from build123d import *

# Parameters (mm, degrees)
SKETCH1_R           = 85
SKETCH1_R_2         = 8.5
BOSS_EXTRUDE1_DEPTH = 10
SKETCH2_R           = 8.5
CUT_EXTRUDE1_DEPTH  = 10
SKETCH4_R           = 5
CUT_EXTRUDE3_DEPTH  = 60


with BuildPart() as part:
    # Sketch1 → Boss-Extrude1 (new body)
    with BuildSketch(Plane.XY):
        Circle(SKETCH1_R)
        Circle(SKETCH1_R_2, mode=Mode.SUBTRACT)
    extrude(amount=BOSS_EXTRUDE1_DEPTH)

    # Sketch2 → Cut-Extrude1 (cut)
    with BuildSketch(Plane.XY.offset(10)):
        with Locations((0, 60)):
            Circle(SKETCH2_R)
        with Locations((57.063390978, 18.541019662)):
            Circle(SKETCH2_R)
        with Locations((35.267115138, -48.541019662)):
            Circle(SKETCH2_R)
        with Locations((-35.267115138, -48.541019662)):
            Circle(SKETCH2_R)
        with Locations((-57.063390978, 18.541019662)):
            Circle(SKETCH2_R)
    extrude(amount=-CUT_EXTRUDE1_DEPTH, mode=Mode.SUBTRACT)

    # Sketch4 → Cut-Extrude3 (cut)
    with BuildSketch(Plane.XY.offset(10)):
        with Locations((0, -48)):
            Circle(SKETCH4_R)
    extrude(amount=-CUT_EXTRUDE3_DEPTH, mode=Mode.SUBTRACT)


solid = part.part
Model file for the job. Use its own axes, mm. Give positions to 0.01 mm unless a question says otherwise; leave off trailing zeros. Order: outer loops, then holes, each group sorted by start corner. A loop starts at its lowest first (then second) coordinate and runs counter-clockwise, first axis right, second up. Notation, with made-up numbers: M -9.5,7.25 L 15.5,7.25 A14 ccw 15.5,16.25 Z; hole C -30.5,-3 d11. An arc over 180 degrees is marked long. Put each result on its own line as item: value. Start each with the question number.
(1) Pin check, flat tips, straight feed: pin 1 Ø1.5 at (y, z) = (36.5, 8.5) entering from +X; pin 2 Ø6 at (y, z) = (37.5, 5.5) entering from -X; pin 3 Ø5 at (x, z) = (46.5, 6.5) entering from +Y. Stop position of each tip, or through.
(2) Band-saw the part on D-D on z = 3. Give the cut face in (x, y).
(3) Band-saw the part on B-B on y = 54. Give the cut face in (x, z), then the cut area to 3 significant figures.
(4) Band-saw the part on A-A on x = 0. Give the cut face in (y, z).
(5) Pull direction Y, two halves, no side cores. Call faces 1 (the face through (-67.453, -51.721, 4.93)), 2 (the face through (-49.21, 15.29, 5.07)), 3 (the face through (18, 1, 0)): released by +Y, released by -Y, zero draft, split by the parting line, or undercut.
(6) Drill centre lines: L1, parallel to Y at x = -0.5, z = 6.75; L2, parallel to Y at x = -32.5, z = 7.25; L3, parallel to X at y = 65, z = 4.25. Where is each one in solid material? Low to high. Write a range as [from, to].
(7) Band-saw the part on C-C on x = 56. Give the cut face in (y, z), then the cut area to 3 significant figures.
Results below:
1. pin 1: stops at x = 77.12
1. pin 2: stops at x = -77.68
1. pin 3: stops at y = 72.73
2. outline: C 0,0 d170; hole C -57.06,18.54 d17; hole C -35.27,-48.54 d17; hole C 0,0 d17; hole C 0,60 d17; hole C 0,-48 d10; hole C 35.27,-48.54 d17; hole C 57.06,18.54 d17
3. outline: M -65.64,0 L -6.02,0 L -6.02,10 L -65.64,10 Z; M 6.02,0 L 65.64,0 L 65.64,10 L 6.02,10 Z
3. area: 1,190 mm2
4. outline: M -85,0 L -53,0 L -53,10 L -85,10 Z; M -43,0 L -8.5,0 L -8.5,10 L -43,10 Z; M 8.5,0 L 51.5,0 L 51.5,10 L 8.5,10 Z; M 68.5,0 L 85,0 L 85,10 L 68.5,10 Z
5. face 1: split by the parting line
5. face 2: undercut
5. face 3: zero draft
6. L1: y = [-85, -52.97], [-43.03, -8.49], [8.49, 51.51], [68.49, 85]
6. L2: y = [-78.54, -56.58], [-40.5, 78.54]
6. L3: x = [-54.77, -6.87], [6.87, 54.77]
7. outline: M -63.95,0 L 10.11,0 L 10.11,10 L -63.95,10 Z; M 26.97,0 L 63.95,0 L 63.95,10 L 26.97,10 Z
7. area: 1,110 mm2
